from build123d import *

# Parameters (mm, degrees)
BOSS_EXTRUDE3_DEPTH = 3


with BuildPart() as part:
    # Sketch1 → Boss-Extrude3 (new body)
    with BuildSketch(Plane.XY):
        Polygon((-61.5, 27.5), (-61.5, 20), (-46.5, 20), (-46.5, -20), (-61.5, -20), (-61.5, -27.5), (-64.5, -27.5), (-64.5, -37.5), (-61.5, -37.5), (-61.5, -42.5), (61.5, -42.5), (61.5, -37.5), (64.5, -37.5), (64.5, -27.5), (61.5, -27.5), (61.5, -20), (46.5, -20), (46.5, 20), (61.5, 20), (61.5, 27.5), (64.5, 27.5), (64.5, 37.5), (61.5, 37.5), (61.5, 42.5), (-61.5, 42.5), (-61.5, 37.5), (-64.5, 37.5), (-64.5, 27.5), align=None)
        with BuildLine():
            Line((-24, 28.5), (24, 28.5))
            ThreePointArc((24, 28.5), (27.5, 25), (24, 21.5))
            Line((24, 21.5), (-24, 21.5))
            ThreePointArc((-24, 21.5), (-27.5, 25), (-24, 28.5))
        make_face(mode=Mode.SUBTRACT)
        with BuildLine():
            Line((-24, -21.5), (24, -21.5))
            ThreePointArc((24, -21.5), (27.5, -25), (24, -28.5))
            Line((24, -28.5), (-24, -28.5))
            ThreePointArc((-24, -28.5), (-27.5, -25), (-24, -21.5))
        make_face(mode=Mode.SUBTRACT)
    extrude(amount=BOSS_EXTRUDE3_DEPTH)


solid = part.part
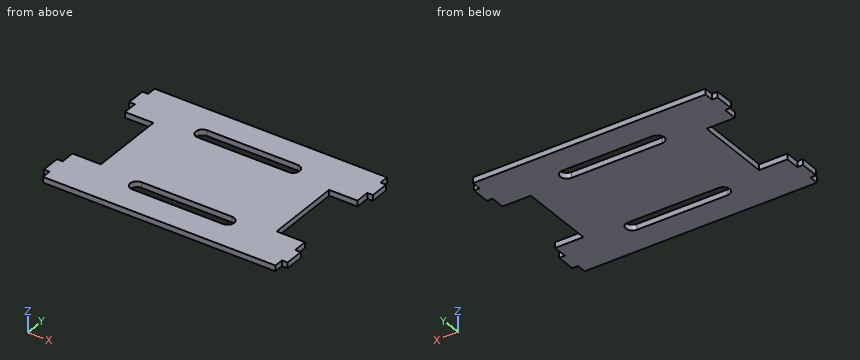
For this review, take the finished solid that the model builds, in its own axes (mm). Coordinates: 2 decimals unless noted, no trailing zeros. Order: outer loops, then holes, each group sorted by start corner. A loop starts at its lowest first (then second) coordinate and runs counter-clockwise, first axis right, second up. Notation, with made-up numbers: (-23.5, -31) - (19.5, -31) arc R18 ccw to (19.5, 2) - close; hole circle Ø10 at (79, 55). An arc over 180 degrees is marked (long way). Answer as CSV lines item,"result". Start each with the question number.
1) Add section D-D (z = 2.55). Count the separate pieces of the cut face and the enclosed holes in it, then the cut area to 3 significant figures.
2) Insertion check: P1, Ø1.5, axis at y = -25, z = 1.5, coming from the +X side; P2, Ø0.9, axis at x = -63.5, z = 1, coming from the +Y side; P3, Ø1.5, axis at y = 1, z = 0.5, coming from the -X side. Each pin has a flat end and moves straight along its axis. Give the tip position at first contact, or say it passes through.
3) Add section C-C (y = 25). State the section outline as (x, z) points.
4) To check wall thickness, follow line 1 along Y through (x, z) = (-13, 1.6); line 2 along Y through (x, z) = (55.5, 0.3); line 3 along X through (y, z) = (5, 0.6). State the ranges of each line that lie inside material, in increasing order. Write a range as [from, to].
5) Add section B-B (x = 50). State the section outline as (y, z) points, then the cut area to 3 significant figures.
6) Add section A-A (x = -16.5). State the section outline as (y, z) points.
Result:
1,separate pieces,"1"
1,enclosed holes,"2"
1,area,"8,630 mm^2"
2,P1,"x = 61.5"
2,P2,"y = 37.5"
2,P3,"x = -46.5"
3,outline,"(-61.5, 0) - (-27.5, 0) - (-27.5, 3) - (-61.5, 3) - close; (27.5, 0) - (61.5, 0) - (61.5, 3) - (27.5, 3) - close"
4,line 1,"[-42.5, -28.5], [-21.5, 21.5], [28.5, 42.5]"
4,line 2,"[-42.5, -20], [20, 42.5]"
4,line 3,"[-46.5, 46.5]"
5,outline,"(-42.5, 0) - (-20, 0) - (-20, 3) - (-42.5, 3) - close; (20, 0) - (42.5, 0) - (42.5, 3) - (20, 3) - close"
5,area,"135 mm^2"
6,outline,"(-42.5, 0) - (-28.5, 0) - (-28.5, 3) - (-42.5, 3) - close; (-21.5, 0) - (21.5, 0) - (21.5, 3) - (-21.5, 3) - close; (28.5, 0) - (42.5, 0) - (42.5, 3) - (28.5, 3) - close"
